Read the model definition and answer for the solid it produces. Units are mm, in the model's axes. Coordinates: 2 decimals unless noted, no trailing zeros. Order: outer loops, then holes, each group sorted by start corner. A loop starts at its lowest first (then second) coordinate and runs counter-clockwise, first axis right, second up. Notation, with made-up numbers: M 72,-13.5 L 80,-13.5 A25 ccw 80,15.5 Z; hole C 9.25,-3.75 d4. An arc over 180 degrees is marked long. Write each question's results on one line, items separated by ' | '.
```python
from build123d import *

# Parameters (mm, degrees)
SKETCH_W    = 105
SKETCH_H    = 85
SKETCH_R    = 2.5
PAD_DEPTH   = 3
FILLET_R    = 1
FILLET001_R = 1


with BuildPart() as part:
    # Sketch → Pad (new body)
    with BuildSketch(Plane.XY):
        Rectangle(SKETCH_W, SKETCH_H)
        with Locations((-46.5, 38)):
            Circle(SKETCH_R, mode=Mode.SUBTRACT)
        with Locations((46.5, 38)):
            Circle(SKETCH_R, mode=Mode.SUBTRACT)
        with Locations((-46.5, -38)):
            Circle(SKETCH_R, mode=Mode.SUBTRACT)
        with Locations((46.5, -38)):
            Circle(SKETCH_R, mode=Mode.SUBTRACT)
    extrude(amount=PAD_DEPTH)

    # Fillet
    fillet_edges = [part.edges().sort_by_distance(p)[0] for p in [
        (52.5, 42.5, 1.5),
    ]]
    fillet(fillet_edges, radius=FILLET_R)

    # Fillet001
    fillet001_edges = [part.edges().sort_by_distance(p)[0] for p in [
        (-52.5, 42.5, 1.5),
        (52.5, -42.5, 1.5),
        (-52.5, -42.5, 1.5),
    ]]
    fillet(fillet001_edges, radius=FILLET001_R)


solid = part.part
```
(1) The part is cut by section B-B, the plane y = -38. Write down the section's boundary in (x, z).
Conclusion:
outline: M -52.5,0 L -49,0 L -49,3 L -52.5,3 Z; M -44,0 L 44,0 L 44,3 L -44,3 Z; M 49,0 L 52.5,0 L 52.5,3 L 49,3 Z
(2) The part is cut by section A-A, the plane x = -46.5. Write down the section's boundary in (y, z), then the cut area to 3 significant figures.
Conclusion:
outline: M -42.5,0 L -40.5,0 L -40.5,3 L -42.5,3 Z; M -35.5,0 L 35.5,0 L 35.5,3 L -35.5,3 Z; M 40.5,0 L 42.5,0 L 42.5,3 L 40.5,3 Z | area: 225 mm²
(3) Straight lines are drawn through the part: line 1 (Y direction, x = 46.5, z = 2.1); line 2 (X direction, y = -36, z = 2.85); line 3 (X direction, y = 36.5, z = 1.6). For each, find the intervals that lie inside material, in ascending order.
Conclusion:
line 1: -42.5 to -40.5, -35.5 to 35.5, 40.5 to 42.5 | line 2: -52.5 to -48, -45 to 45, 48 to 52.5 | line 3: -52.5 to -48.5, -44.5 to 44.5, 48.5 to 52.5
(4) The mould has two halves that part along Y. Classify faces 1 (the flat face through (52.5, -1, 1)), 2 (the flat face through (-1, -42.5, 1)), 3 (the cylindrical face through (-44.19, -38.96, 1.48)), 4 (the cylindrical face through (48.81, 37.04, 1.48)): pulls with the +Y half, pulls with the -Y half, needs draft (parallel to the pull), parting line crosses it, or undercut.
Conclusion:
face 1: needs draft | face 2: pulls with the -Y half | face 3: undercut | face 4: undercut
